Work out the finished part from the listing and answer in its coordinate system (mm). Face numbers are marked on the shaded views. A direction names the side the tool comes from. Round coordinates to 2 decimals unless told otherwise and drop trailing zeros. Order: outer loops, then holes, each group sorted by start corner. A loop starts at its lowest first (then second) coordinate and runs counter-clockwise, first axis right, second up.
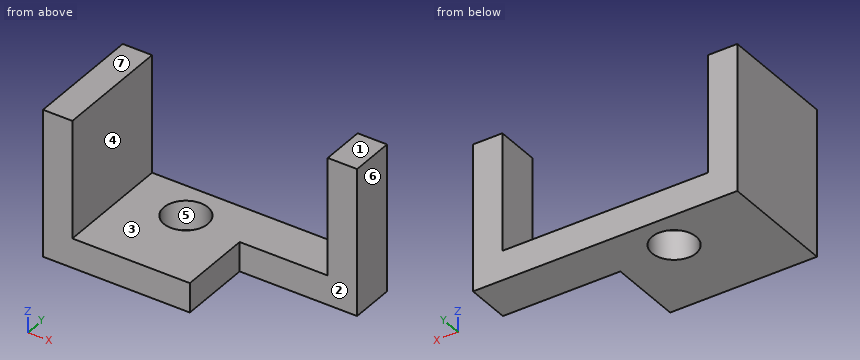
from build123d import *

# Parameters (mm, degrees)
F1_DEPTH = 20
F0_W     = 20
F0_H     = 80
F0_H_2   = 30
F2_DEPTH = 100
F4_D     = 30


with BuildPart() as f1:
    # F0 (on Top) → F1 (new body)
    with BuildSketch(Plane.XY):
        Polygon((111.985649, 39.813087), (-28.014351, 39.813087), (-28.014351, -40.186913), (51.985649, -40.186913), (51.985649, 9.813087), (111.985649, 9.813087), align=None)
    extrude(amount=F1_DEPTH)

    # F0 (on Top) → F2 (join)
    with BuildSketch(Plane.XY):
        with Locations((-38.014351, -0.186913)):
            Rectangle(F0_W, F0_H)
        with Locations((121.985649, 24.813087)):
            Rectangle(F0_W, F0_H_2)
    extrude(amount=F2_DEPTH)

    # F4 (through all)
    with Locations(Plane.XY.offset(20)):
        with Locations((11.985649, 14.813087)):
            Hole(F4_D / 2)


solid = f1.part
Item 1: For a pull along X with two mould halves and no side action, classify the marked faces 4, 5, 6 and 7 as released by +X, released by -X, zero draft, split by the parting line, or undercut.
Item 2: Find section D-D (y = -3). Write down the section's boundary in (x, z), plus the area to 3 significant figures.
Item 3: Given pin 1 (8 mm diameter, centred on x = 64.5, y = 9, fed in from +Z); pin 2 (1 mm diameter, centred on x = -17, y = -23, fed in from -Z); pin 3 (24 mm diameter, centred on y = -10.5, z = 64, fed in from +X); pin 4 (6 mm diameter, centred on y = -12.5, z = 12.5, fed in from +X), each flat-ended and moving along its own axis, determine where each tip first touches the part or whether it passes through.
Item 4: Find section B-B (y = 7.5). Write down the section's boundary in (x, z).
Item 5: Find section C-C (x = 9). Write down the section's boundary in (y, z).
Item 6: A tool of negligible diameter and unlimited length cuts with its end or side. For the marked faces 1, 2 and 3, from which of +Z, -Z, +X, -X, +Y, -Y can it reach the whole face along a straight path? Write none if from no direction.
Item 7: Find section A-A (z = 54.5). Write down the section's boundary in (x, y).
Item 8: Find the intervals of material crossed by line 1 along X through (y, z) = (25.5, 86); line 2 along X through (y, z) = (-2, 6.5); line 3 along Z through (x, y) = (90, 12), in increasing order.
Model answer:
1. face 4: undercut
1. face 5: undercut
1. face 6: released by +X
1. face 7: zero draft
2. outline: (-48.01, 0) - (51.99, 0) - (51.99, 20) - (-28.01, 20) - (-28.01, 100) - (-48.01, 100) - close
2. area: 3,600 mm2
3. pin 1: stops at z = 20
3. pin 2: stops at z = 0
3. pin 3: stops at x = -28.01
3. pin 4: stops at x = 51.99
4. outline: (-48.01, 0) - (-1.11, 0) - (-1.11, 20) - (-28.01, 20) - (-28.01, 100) - (-48.01, 100) - close; (25.08, 0) - (51.99, 0) - (51.99, 20) - (25.08, 20) - close
5. outline: (-40.19, 0) - (0.11, 0) - (0.11, 20) - (-40.19, 20) - close; (29.51, 0) - (39.81, 0) - (39.81, 20) - (29.51, 20) - close
6. face 1: +Z, +X, -X, +Y, -Y
6. face 2: +Z, -Z, +X, -Y
6. face 3: +Z, +Y, -Y
7. outline: (-48.01, -40.19) - (-28.01, -40.19) - (-28.01, 39.81) - (-48.01, 39.81) - close; (111.99, 9.81) - (131.99, 9.81) - (131.99, 39.81) - (111.99, 39.81) - close
8. line 1: x = -48.01 to -28.01, 111.99 to 131.99
8. line 2: x = -48.01 to 51.99
8. line 3: z = 0 to 20
